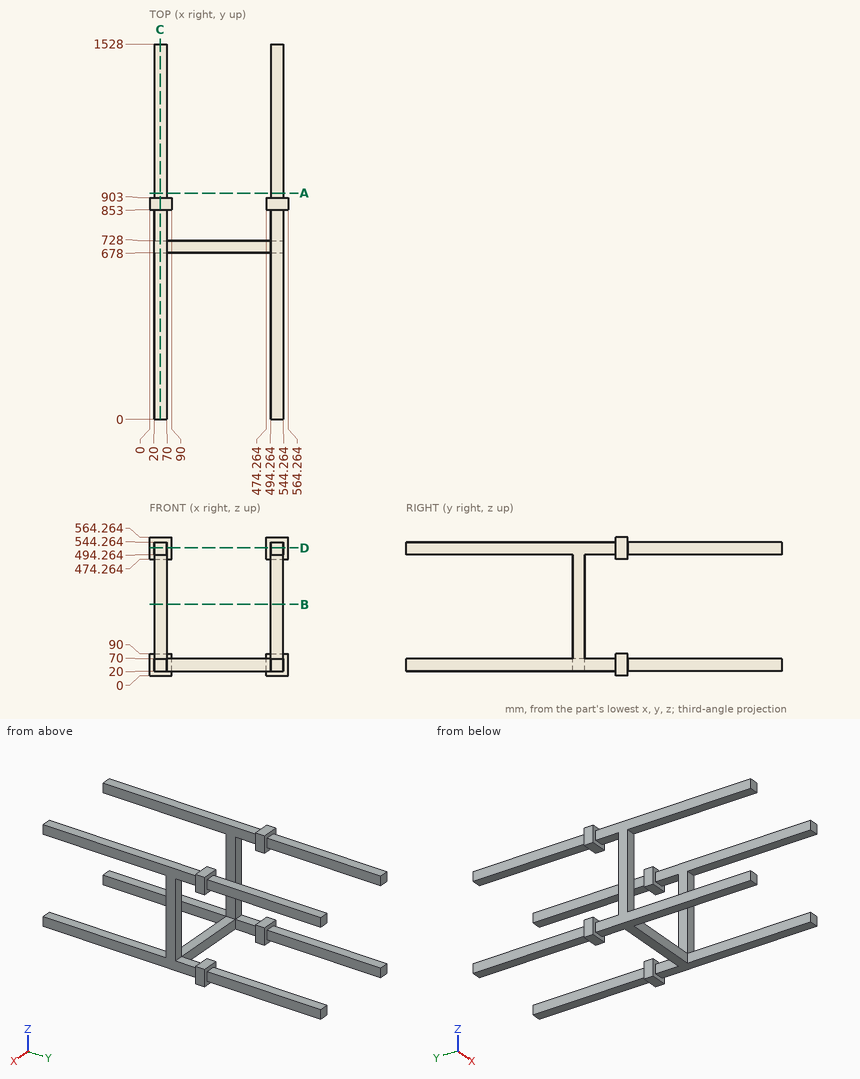
Could you check a few things on this drawing? It's one solid part, dimensions in mm from its lowest x, y, z. Coordinates: 2 decimals unless noted, no trailing zeros. Order: outer loops, then holes, each group sorted by start corner. A loop starts at its lowest first (then second) coordinate and runs counter-clockwise, first axis right, second up.
1) Imagine slicing it at D-D on z = 521.5. List the corners of the cut face in (x, y) for me, and give its area (3 significant figures).
2) Imagine slicing it at A-A on y = 921. List the corners of the cut face in (x, z) for me, and give its area (3 significant figures).
3) Imagine slicing it at B-B on z = 292. List the corners of the cut face in (x, y) for me, and give its area (3 significant figures).
4) Will these pins go through, and if not, where does the flat tip stop? pin 1 (3 mm diameter, centred on x = 86, z = 496, fed in from -Y); pin 2 (25 mm diameter, centred on x = 513, y = 318.5, fed in from -Z); pin 3 (1 mm diameter, centred on y = 1230.5, z = 499, fed in from -X).
5) I need wall thicknesses on line 1 (X direction, y = 725, z = 125); line 2 (Y direction, x = 504.5, z = 483.5). Which ranges of each line are inside material? Lowest first, please.
6) Imagine slicing it at C-C on x = 43.5. List the corners of the cut face in (y, z) for me.
Response values:
1. outline: (0, 853) - (20, 853) - (20, 0) - (70, 0) - (70, 853) - (90, 853) - (90, 903) - (70, 903) - (70, 1528) - (20, 1528) - (20, 903) - (0, 903) - close; (474.26, 853) - (494.26, 853) - (494.26, 0) - (544.26, 0) - (544.26, 853) - (564.26, 853) - (564.26, 903) - (544.26, 903) - (544.26, 1528) - (494.26, 1528) - (494.26, 903) - (474.26, 903) - close
1. area: 157,000 mm2
2. outline: (20, 20) - (70, 20) - (70, 70) - (20, 70) - close; (20, 494.26) - (70, 494.26) - (70, 544.26) - (20, 544.26) - close; (494.26, 20) - (544.26, 20) - (544.26, 70) - (494.26, 70) - close; (494.26, 494.26) - (544.26, 494.26) - (544.26, 544.26) - (494.26, 544.26) - close
2. area: 10,000 mm2
3. outline: (20, 678) - (70, 678) - (70, 728) - (20, 728) - close; (494.26, 678) - (544.26, 678) - (544.26, 728) - (494.26, 728) - close
3. area: 5,000 mm2
4. pin 1: stops at y = 853
4. pin 2: stops at z = 20
4. pin 3: stops at x = 20
5. line 1: x = 20 to 70, 494.26 to 544.26
5. line 2: y = 678 to 728, 853 to 903
6. outline: (0, 20) - (853, 20) - (853, 0) - (903, 0) - (903, 20) - (1528, 20) - (1528, 70) - (903, 70) - (903, 90) - (853, 90) - (853, 70) - (728, 70) - (728, 494.26) - (853, 494.26) - (853, 474.26) - (903, 474.26) - (903, 494.26) - (1528, 494.26) - (1528, 544.26) - (903, 544.26) - (903, 564.26) - (853, 564.26) - (853, 544.26) - (0, 544.26) - (0, 494.26) - (678, 494.26) - (678, 70) - (0, 70) - close
